```python
from build123d import *

# Parameters (mm, degrees)
SKETCH_1_W      = 12.4
SKETCH_1_H      = 22.3
EXTRUDE_1_DEPTH = 22.6
EXTRUDE_2_DEPTH = 4.3
SKETCH_3_R      = 2.5
EXTRUDE_3_DEPTH = 9.3
EXTRUDE_4_DEPTH = 2.4
SKETCH_5_R      = 0.6
EXTRUDE_5_DEPTH = 2.3


with BuildPart() as part:
    # 草图1 → 凸台-拉伸1 (new body)
    with BuildSketch(Plane.XY):
        Rectangle(SKETCH_1_W, SKETCH_1_H)
    extrude(amount=EXTRUDE_1_DEPTH)

    # 草图2 → 凸台-拉伸2 (add)
    with BuildSketch(Plane(origin=(0, 11.15, 0), x_dir=(1, 0, 0), z_dir=(0, 1, 0))):
        with BuildLine():
            ThreePointArc((1.29283601, -12.263709677), (0, 0), (-1.29283601, -12.263709677))
            ThreePointArc((-1.29283601, -12.263709677), (0, -13.7), (1.29283601, -12.263709677))
        make_face()
    extrude(amount=EXTRUDE_2_DEPTH)

    # 草图3 → 凸台-拉伸3 (add)
    with BuildSketch(Plane(origin=(0, 15.45, 0), x_dir=(1, 0, 0), z_dir=(0, 1, 0))):
        with Locations(Location((0, -6.2, 0), (0, 0, 270))):
            Circle(SKETCH_3_R)
    extrude(amount=EXTRUDE_3_DEPTH)

    # 草图4 → 凸台-拉伸4 (add)
    with BuildSketch(Plane(origin=(0, 9.3, 0), x_dir=(1, 0, 0), z_dir=(0, 1, 0))):
        with BuildLine():
            Line((6.2, -22.6), (-6.2, -22.6))
            Line((-6.2, -22.6), (-6.2, -27.6))
            Line((-6.2, -27.6), (-0.55, -27.6))
            Line((-0.55, -27.6), (-0.55, -25.935164654))
            ThreePointArc((-0.55, -25.935164654), (0, -24.1), (0.55, -25.935164654))
            Line((0.55, -25.935164654), (0.55, -27.6))
            Line((0.55, -27.6), (6.2, -27.6))
            Line((6.2, -27.6), (6.2, -22.6))
        make_face()
        with BuildLine():
            Line((0.55, 3.035164654), (0.55, 4.7))
            Line((0.55, 4.7), (6.2, 4.7))
            Line((6.2, 4.7), (6.2, -0.3))
            Line((6.2, -0.3), (-6.2, -0.3))
            Line((-6.2, -0.3), (-6.2, 4.7))
            Line((-6.2, 4.7), (-0.55, 4.7))
            Line((-0.55, 4.7), (-0.55, 3.035164654))
            ThreePointArc((-0.55, 3.035164654), (0, 1.2), (0.55, 3.035164654))
        make_face()
    extrude(amount=-EXTRUDE_4_DEPTH)

    # 草图5 → 凸台-拉伸5 (add)
    with BuildSketch(Plane(origin=(0, 0, 0), x_dir=(-1, 0, 0), z_dir=(0, 0, -1))):
        with Locations((0, -6.65)):
            Circle(SKETCH_5_R)
        with Locations((-1.21, -6.65)):
            Circle(SKETCH_5_R)
        with Locations((1.21, -6.65)):
            Circle(SKETCH_5_R)
    extrude(amount=EXTRUDE_5_DEPTH)


solid = part.part
```
Work out the finished part from the listing and answer in its coordinate system (mm). A direction names the side the tool comes from. Give positions to 0.01 mm unless a question says otherwise; leave off trailing zeros. Loops run counter-clockwise (first coordinate to the right, second up) from the corner with the lowest first, then second, coordinate; pieces in that order, holes last. Notation, with made-up numbers: (54.25, -38) - (66.25, -38) arc R25 cw to (66.25, 0) - close; hole circle Ø7 at (34, 44). An arc over 180 degrees is marked (long way). Use CSV: the item, a comma, the result in double quotes. Start each with the question number.
(1) Find the intervals of material crossed by L1, parallel to X at y = 8, z = 25; L2, parallel to Y at x = 5, z = 18.5; L3, parallel to Y at x = -1.5, z = -1, in increasing order.
(2) Find section A-A, the plane z = -0.5. Determine the outline of the cut face in (x, y).
(3) A tool of negligible diameter and unlimited length cuts with its end or side. For faces 4 (the face through (1.5, 6.9, -2.4)), 5 (the face through (0.55, 8, 27)), 6 (the face through (3, 15.45, 7)), from which of +Z, -Z, +X, -X, +Y, -Y can it reach the whole face along a straight path? Write none if from no direction.
(4) Find section B-B, the plane z = 25.1. Determine the outline of the cut face in (x, y), plus the area to 3 significant figures.
(5) Each of these flat-tipped pins is pushed along its axis until it touches: pin 1 (5 mm diameter, centred on x = 5, z = 23, fed in from +Y); pin 2 (1.2 mm diameter, centred on x = 0, z = -2.2, fed in from -Y); pin 3 (1.4 mm diameter, centred on x = 1.5, z = -3, fed in from +Y); pin 4 (1.8 mm diameter, centred on x = 0, z = 25.1, fed in from -Y). Where does it stop, or does it pass through?
(6) Determine the mould class of faces 1 (the face through (0.55, 8, -4)), 2 (the face through (1, -7, -2.3)), 3 (the face through (0, 8.1, 24.1)) for opening direction Z: released by +Z, released by -Z, zero draft, split by the parting line, or undercut.
(7) Find section D-D, the plane x = -3.75. Determine the outline of the cut face in (y, z).
Results found:
1,L1,"-6.2 to -0.99, 0.99 to 6.2"
1,L2,"-11.15 to 11.15"
1,L3,"-7.18 to -6.12, 6.9 to 9.3"
2,outline,"(-6.2, 6.9) - (6.2, 6.9) - (6.2, 9.3) - (-6.2, 9.3) - close; circle Ø1.2 at (-1.21, -6.65); circle Ø1.2 at (0, -6.65); circle Ø1.2 at (1.21, -6.65)"
3,face 4,"-Z, +X, -X"
3,face 5,"+Z, +Y, -Y"
3,face 6,"+Y"
4,outline,"(-6.2, 6.9) - (-1, 6.9) - (-1, 9.3) - (-6.2, 9.3) - close; (1, 6.9) - (6.2, 6.9) - (6.2, 9.3) - (1, 9.3) - close"
4,area,"25.0 mm^2"
5,pin 1,"y = 11.15"
5,pin 2,"y = -7.25"
5,pin 3,"y = 9.3"
5,pin 4,"through"
6,face 1,"zero draft"
6,face 2,"released by -Z"
6,face 3,"undercut"
7,outline,"(-11.15, 0) - (6.9, 0) - (6.9, -4.7) - (9.3, -4.7) - (9.3, 0) - (11.15, 0) - (11.15, 1.26) - (15.45, 1.26) - (15.45, 11.14) - (11.15, 11.14) - (11.15, 22.6) - (9.3, 22.6) - (9.3, 27.6) - (6.9, 27.6) - (6.9, 22.6) - (-11.15, 22.6) - close"
